Source: CAD feature listing. Evaluate the final solid. Frame: model axes, mm. Coordinates: 2 decimals unless noted, no trailing zeros. Order: outer loops, then holes, each group sorted by start corner. A loop starts at its lowest first (then second) coordinate and runs counter-clockwise, first axis right, second up.
Item 1: Section C-C on x = 115.5. Return the cut outline in (y, z), then the cut area to 3 significant figures.
Item 2: Section B-B on y = 116. Return the cut outline in (x, z), then the cut area to 3 significant figures.
Item 3: Contact query for flat-ended pins moving along their axis: P1, Ø8, axis at x = 32.5, z = 552, coming from the +Y side; P2, Ø7, axis at x = 100.9, y = 60.09, coming from the -Z side; P3, Ø3, axis at x = 68, y = 84, coming from the -Z side; P4, Ø5, axis at x = 47, y = 136.5, coming from the +Z side. Output: stop coordinate, or through.
Item 4: Section A-A on z = 325. Return the cut outline in (x, y).
Item 5: Ray query, line 1 (Y direction, x = 118, z = 160); line 2 (Y direction, x = 112, z = 651); line 3 (X direction, y = 144, z = 600.5). Return the intervals inside material, ascending.
from build123d import *

# Parameters (mm, degrees)
F1_DEPTH       = 711.2
F3_D           = 5.5
F3_DEPTH       = 25.4
F3_CBORE_D     = 9.75
F3_CBORE_DEPTH = 5
F3_TIP         = 1.6523667023


# Not quite as in the source:
# - a feature names something its author has since deleted; it is built from what else it names


with BuildPart() as f1:
    # F0 (on Top) → F1 (new body)
    with BuildSketch(Plane.XY):
        Polygon((0, 101.6), (0, 0), (152.4, 0), (152.4, 101.6), (76.2, 152.4), align=None)
    extrude(amount=F1_DEPTH)

    # F3
    with Locations(Plane(origin=(0, 0, 0), x_dir=(1, 0, 0), z_dir=(0, 0, -1))):
        with Locations((100.9017452598, -60.0949265063), (67.4944594502, -83.0287188292)):
            CounterBoreHole(F3_D / 2, F3_CBORE_D / 2, F3_CBORE_DEPTH, depth=F3_DEPTH)
            with Locations((0, 0, -(F3_DEPTH + F3_TIP / 2))):  # 118° drill point
                Cone(0, F3_D / 2, F3_TIP, mode=Mode.SUBTRACT)


solid = f1.part
Answer list:
1. outline: (0, 0) - (126.2, 0) - (126.2, 711.2) - (0, 711.2) - close
1. area: 89,800 mm2
2. outline: (21.6, 0) - (130.8, 0) - (130.8, 711.2) - (21.6, 711.2) - close
2. area: 77,700 mm2
3. P1: stops at y = 125.93
3. P2: stops at z = 5
3. P3: stops at z = 25.49
3. P4: passes through
4. outline: (0, 0) - (152.4, 0) - (152.4, 101.6) - (76.2, 152.4) - (0, 101.6) - close
5. line 1: y = 0 to 124.53
5. line 2: y = 0 to 128.53
5. line 3: x = 63.6 to 88.8
